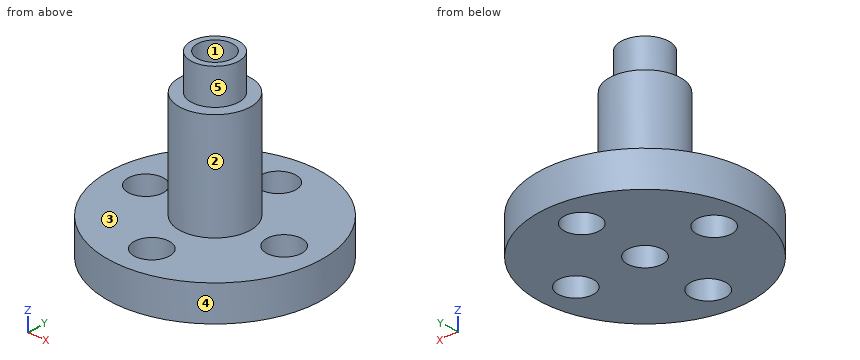
```python
from build123d import *

# Parameters (mm, degrees)
F0_R     = 38.1
F1_DEPTH = 12.7
F2_R     = 6.35
F3_DEPTH = 12.701
F4_R     = 12.7
F5_DEPTH = 38.1
F6_R     = 8.5725
F7_DEPTH = 12.7
F8_R     = 6.35
F9_DEPTH = 63.501


with BuildPart() as f1:
    # F0 (on Top) → F1 (new body)
    with BuildSketch(Plane.XY):
        Circle(F0_R)
    extrude(amount=F1_DEPTH)

    # F2 (on face) → F3 (cut, through all)
    with BuildSketch(Plane.XY.offset(12.7)):
        with Locations((0, 25.4)):
            Circle(F2_R)
        with Locations((25.4, 0)):
            Circle(F2_R)
        with Locations((0, -25.4)):
            Circle(F2_R)
        with Locations((-25.4, 0)):
            Circle(F2_R)
    extrude(amount=-F3_DEPTH, mode=Mode.SUBTRACT)

    # F4 (on face) → F5 (join)
    with BuildSketch(Plane.XY.offset(12.7)):
        Circle(F4_R)
    extrude(amount=F5_DEPTH)

    # F6 (on face) → F7 (join)
    with BuildSketch(Plane.XY.offset(50.8)):
        Circle(F6_R)
    extrude(amount=F7_DEPTH)

    # F8 (on face) → F9 (cut, through all)
    with BuildSketch(Plane.XY.offset(63.5)):
        Circle(F8_R)
    extrude(amount=-F9_DEPTH, mode=Mode.SUBTRACT)


solid = f1.part
```
For this review, take the finished solid that the model builds, in its own axes (mm). Face numbers are marked on the shaded views. A direction names the side the tool comes from. Give positions to 0.01 mm unless a question says otherwise; leave off trailing zeros. Write each loop counter-clockwise with the first axis right and the second up, starting at its lowest first coordinate (ties: lowest second). Pieces come first, ordered by that corner, then holes. Notation, with made-up numbers: M 85.5,54.25 L 96.5,54.25 A22 ccw 96.5,80.25 Z; hole C 8.5,27.25 d10. An arc over 180 degrees is marked long. Answer as CSV lines item,"result".
1. Wall thickness on line 1 (Y direction, x = 0, z = 5.75); line 2 (Z direction, x = 18.5, y = 4); line 3 (Y direction, x = -25, z = 6): over which ranges is each line inside the solid? List them lowest first.
Findings:
line 1,"y = -38.1 to -31.75, -19.05 to -6.35, 6.35 to 19.05, 31.75 to 38.1"
line 2,"z = 0 to 12.7"
line 3,"y = -28.75 to -6.34, 6.34 to 28.75"
2. For pin 1 (10 mm diameter, centred on x = 5, z = 22.5, fed in from -Y); pin 2 (1.5 mm diameter, centred on x = -8.5, z = 14.5, fed in from -Y); pin 3 (1.5 mm diameter, centred on y = -4, z = 42.5, fed in from -X), all flat-tipped, find the tip position at first contact; note any pin that passes through.
Findings:
pin 1,"stops at y = -12.7"
pin 2,"stops at y = -10.06"
pin 3,"stops at x = -12.28"
3. Consider section A-A, the plane y = 0. Write out the cut boundary in (x, z), then the cut area to 3 significant figures.
Findings:
outline,"M -38.1,0 L -31.75,0 L -31.75,12.7 L -38.1,12.7 Z; M -19.05,0 L -6.35,0 L -6.35,63.5 L -8.57,63.5 L -8.57,50.8 L -12.7,50.8 L -12.7,12.7 L -19.05,12.7 Z; M 6.35,0 L 19.05,0 L 19.05,12.7 L 12.7,12.7 L 12.7,50.8 L 8.57,50.8 L 8.57,63.5 L 6.35,63.5 Z; M 31.75,0 L 38.1,0 L 38.1,12.7 L 31.75,12.7 Z"
area,"1,020 mm2"
4. For the marked faces 4 and 5, list the 3-axis set-ups (+Z, -Z, +X, -X, +Y, -Y) from which the entire face can be reached by the end or side of a thin tool; tool diameter is ignored.
Findings:
face 4,"+Z, -Z"
face 5,"+Z"
5. Draft analysis for pull direction X (two halves, no side actions). For the marked faces 1, 2 and 3, state which applies: +X half, -X half, draft (parallel to the pull), parting line (faces both ways), or undercut.
Findings:
face 1,"undercut"
face 2,"parting line"
face 3,"draft"
6. Consider section C-C, the plane x = -25.4. Write out the cut boundary in (y, z), then the cut area to 3 significant figures.
Findings:
outline,"M -28.4,0 L -6.35,0 L -6.35,12.7 L -28.4,12.7 Z; M 6.35,0 L 28.4,0 L 28.4,12.7 L 6.35,12.7 Z"
area,"560 mm2"
